Can you work these out from the model? Positions are in its coordinate system, mm. A direction names the side the tool comes from. Coordinates: 2 decimals unless noted, no trailing zeros. Write each loop counter-clockwise with the first axis right and the second up, starting at its lowest first coordinate (ties: lowest second). Pieces come first, ordered by that corner, then holes. Notation, with made-up numbers: (14.25, 45) - (68.25, 45) arc R34 cw to (68.25, 75) - close; hole circle Ø1 at (43, 60.5). An arc over 180 degrees is marked (long way). Use one line per item in the form item = value. Start each with the question number.
(1) If we section it at C-C on x = 9.25: Please give me the cut outline in (y, z).
(2) If I drill on probe 1 along Y at (x, z) = (0, -0.7); probe 2 along Y at (x, z) = (0, 1.95); probe 3 along Z at (x, y) = (-7.5, 7), over which ranges is the centre line in solid material (lowest first)? Write a range as from..to.
(3) If we section it at A-A on y = -1.5: Please give me the cut outline in (x, z), then the cut area to 3 significant figures.
(4) If we section it at B-B on x = 1.75: Please give me the cut outline in (y, z).
(5) Thinking about a two-plate mould opening in X: for faces 1 (the face through (-6.4, 12, 0)), 2 (the face through (0.3, 11.484, 0.02)), 3 (the face through (6.448, 11.909, 0.029)), 4 (the face through (0, 9, 2.05)), which applies, pulls with the +X half, pulls with the -X half, needs draft (parallel to the pull), parting line crosses it, or undercut?
(6) On a 3-axis mill with a long thin cutter (end or side, diameter ignored), from which of +Z, -Z, +X, -X, +Y, -Y can I reach the whole of each face in a straight line? I mean faces 5 (the face through (-11, -5, 0)), 6 (the face through (0, 9, -2.05)), 7 (the face through (0.332, 6.995, 1.73)), 8 (the face through (6, 15, 0)), 9 (the face through (-6, 15, 0)). Say none if no direction works.
(7) For pin 1 Ø6 at (x, y) = (1.5, 2) entering from -Z; pin 2 Ø1.4 at (y, z) = (-4.5, 0.5) entering from -X; pin 3 Ø0.9 at (y, z) = (15, 0) entering from +X; pin 4 Ø7 at (x, y) = (0, 17.03) entering from -Z, each with a flat end and sliding along its axis, tell me the tip position at first contact or that it passes through.
```python
from build123d import *

# Parameters (mm, degrees)
F0_R     = 2.7
F1_DEPTH = 2.05
F2_R     = 5.99999
F3_R     = 4
F4_R     = 10.5
F5_DEPTH = 4.101
F7_DEPTH = 1.4


# Not quite as in the source:
# - a fillet or chamfer is up to 0.001 mm smaller than in the source, because OpenCascade refuses the exact size


with BuildPart() as f1:
    # F0 (on Top) → F1 (new body, symmetric)
    with BuildSketch(Plane.XY):
        with BuildLine():
            ThreePointArc((-6, 11.5325625947), (-6.7453687816, -11.1130553854), (13, 0))
            ThreePointArc((13, 0), (11.1130553854, 6.7453687816), (6, 11.5325625947))
            Line((6, 11.5325625947), (-6, 11.5325625947))
        make_face()
        with BuildLine():
            Line((-6, 11.5325625947), (6, 11.5325625947))
            ThreePointArc((6, 11.5325625947), (0, 13), (-6, 11.5325625947))
        make_face()
        with BuildLine():
            ThreePointArc((-6, 11.5325625947), (0, 13), (6, 11.5325625947))
            Line((6, 11.5325625947), (6, 21.5325625947))
            Line((6, 21.5325625947), (-6, 21.5325625947))
            Line((-6, 21.5325625947), (-6, 11.5325625947))
        make_face()
        with Locations((0, 17.0325625947)):
            Circle(F0_R, mode=Mode.SUBTRACT)
    extrude(amount=F1_DEPTH, both=True)

    # F2 (radius 6 in the source; OpenCascade refuses exactly that, so slightly less here)
    f2_edges = [f1.edges().sort_by_distance(p)[0] for p in [
        (-6, 21.532563, 0),
        (6, 21.532563, 0),
    ]]
    fillet(f2_edges, radius=F2_R)

    # F3
    f3_edges = [f1.edges().sort_by_distance(p)[0] for p in [
        (6, 11.532563, 0),
        (-6, 11.532563, 0),
    ]]
    fillet(f3_edges, radius=F3_R)

    # F4 (on face) → F5 (cut, through all)
    with BuildSketch(Plane.XY.offset(2.05)):
        with Locations((0, -3.5)):
            Circle(F4_R)
    extrude(amount=-F5_DEPTH, mode=Mode.SUBTRACT)

    # F6 (on Top) → F7 (cut, symmetric)
    with BuildSketch(Plane.XY):
        with BuildLine():
            ThreePointArc((11, -3.3115318698), (11.3650882253, -1.6736227042), (11.4876561284, 0))
            ThreePointArc((11.4876561284, 0), (-1.6736227042, 11.3650882253), (-11, -3.3115318698))
            Line((-11, -3.3115318698), (11, -3.3115318698))
        make_face()
        with BuildLine():
            Line((11, -3.3115318698), (-11, -3.3115318698))
            ThreePointArc((-11, -3.3115318698), (0, -11.4876561284), (11, -3.3115318698))
        make_face()
        with BuildLine():
            ThreePointArc((11, -3.3115318698), (0, -11.4876561284), (-11, -3.3115318698))
            Line((-11, -3.3115318698), (-11, -30.7711608721))
            Line((-11, -30.7711608721), (11, -30.7711608721))
            Line((11, -30.7711608721), (11, -3.3115318698))
        make_face()
    extrude(amount=F7_DEPTH, both=True, mode=Mode.SUBTRACT)


solid = f1.part
```
Reported:
q1.outline = (-9.13, -2.05) - (-8.47, -2.05) - (-8.47, -1.4) - (-9.13, -1.4) - close; (-9.13, 1.4) - (-8.47, 1.4) - (-8.47, 2.05) - (-9.13, 2.05) - close; (1.47, -2.05) - (9.13, -2.05) - (9.13, 2.05) - (1.47, 2.05) - (1.47, 1.4) - (6.81, 1.4) - (6.81, -1.4) - (1.47, -1.4) - close
q2.probe_1 = 11.49..14.33, 19.73..21.53
q2.probe_2 = 7..14.33, 19.73..21.53
q2.probe_3 = -2.05..-1.4, 1.4..2.05
q3.outline = (-12.91, -2.05) - (-10.31, -2.05) - (-10.31, -1.4) - (-11.39, -1.4) - (-11.39, 1.4) - (-10.31, 1.4) - (-10.31, 2.05) - (-12.91, 2.05) - close; (10.31, -2.05) - (12.91, -2.05) - (12.91, 2.05) - (10.31, 2.05) - (10.31, 1.4) - (11.39, 1.4) - (11.39, -1.4) - (10.31, -1.4) - close
q3.area = 15.3 mm2
q4.outline = (6.85, -2.05) - (14.98, -2.05) - (14.98, 2.05) - (6.85, 2.05) - (6.85, 1.4) - (11.35, 1.4) - (11.35, -1.4) - (6.85, -1.4) - close; (19.09, -2.05) - (21.27, -2.05) - (21.27, 2.05) - (19.09, 2.05) - close
q5.face_1 = pulls with the -X half
q5.face_2 = undercut
q5.face_3 = pulls with the +X half
q5.face_4 = needs draft
q6.face_5 = -Y
q6.face_6 = -Z, +X, -X, +Y, -Y
q6.face_7 = +Z, -Z
q6.face_8 = +Z, -Z, +X, +Y
q6.face_9 = +Z, -Z, -X, +Y
q7.pin_1 = through
q7.pin_2 = -12.43
q7.pin_3 = 6
q7.pin_4 = -2.05
